Could you check a few things on this model? Use its own coordinates, in mm. A direction names the side the tool comes from. Round coordinates to 2 decimals unless told otherwise and drop trailing zeros. Loops run counter-clockwise (first coordinate to the right, second up) from the corner with the lowest first, then second, coordinate; pieces in that order, holes last. Notation, with made-up numbers: (89, 42.25) -> (124, 42.25) arc R28 cw to (124, 78.25) -> close; hole circle Ø4 at (3.5, -9.5). An arc over 180 degrees is marked (long way). One line per item, written item: value.
from build123d import *

# Parameters (mm, degrees)
F0_R     = 10.5
F0_W     = 6
F0_H     = 27
F0_W_2   = 3
F1_DEPTH = 3
F2_DEPTH = 22
F3_R     = 2.99999
F5_R     = 10.5
F6_DEPTH = 12
F7_DEPTH = 3
F8_R     = 5


# Not quite as in the source:
# - a fillet or chamfer is up to 0.001 mm smaller than in the source, because OpenCascade refuses the exact size


with BuildPart() as f1:
    # F0 (on Top) → F1 (new body)
    with BuildSketch(Plane.XY):
        with BuildLine():
            ThreePointArc((0, -13.5), (9.545941546, -9.545941546), (13.5, 0))
            ThreePointArc((13.5, 0), (9.545941546, 9.545941546), (0, 13.5))
            ThreePointArc((0, 13.5), (-13.5, 0), (0, -13.5))
        make_face()
        Circle(F0_R, mode=Mode.SUBTRACT)
        with BuildLine():
            Line((13.5, -13.5), (13.5, 0))
            ThreePointArc((13.5, 0), (9.545941546, -9.545941546), (0, -13.5))
            Line((0, -13.5), (13.5, -13.5))
        make_face()
        with BuildLine():
            ThreePointArc((0, 13.5), (9.545941546, 9.545941546), (13.5, 0))
            Line((13.5, 0), (13.5, 13.5))
            Line((13.5, 13.5), (0, 13.5))
        make_face()
        Polygon((13.5, 13.5), (13.5, 0), (13.5, -13.5), (16.5, -13.5), (16.5, 13.5), align=None)
        with Locations((19.5, 0)):
            Rectangle(F0_W, F0_H)
        with Locations((24, 0)):
            Rectangle(F0_W_2, F0_H)
    extrude(amount=F1_DEPTH)

    # F0 (on Top) → F2 (join)
    with BuildSketch(Plane.XY):
        with BuildLine():
            ThreePointArc((0, -13.5), (9.545941546, -9.545941546), (13.5, 0))
            ThreePointArc((13.5, 0), (9.545941546, 9.545941546), (0, 13.5))
            ThreePointArc((0, 13.5), (-13.5, 0), (0, -13.5))
        make_face()
        Circle(F0_R, mode=Mode.SUBTRACT)
        with BuildLine():
            ThreePointArc((0, 13.5), (9.545941546, 9.545941546), (13.5, 0))
            Line((13.5, 0), (13.5, 13.5))
            Line((13.5, 13.5), (0, 13.5))
        make_face()
        Polygon((13.5, 13.5), (13.5, 0), (13.5, -13.5), (16.5, -13.5), (16.5, 13.5), align=None)
        with Locations((24, 0)):
            Rectangle(F0_W_2, F0_H)
        with BuildLine():
            Line((13.5, -13.5), (13.5, 0))
            ThreePointArc((13.5, 0), (9.545941546, -9.545941546), (0, -13.5))
            Line((0, -13.5), (13.5, -13.5))
        make_face()
    extrude(amount=-F2_DEPTH)

    # F3 (radius 3 in the source; OpenCascade refuses exactly that, so slightly less here)
    f3_edges = [f1.edges().sort_by_distance(p)[0] for p in [
        (16.5, 0, 0),
        (22.5, 0, 0),
        (25.5, 0, 3),
    ]]
    fillet(f3_edges, radius=F3_R)



with BuildPart() as f6:
    # F5 (on offset) → F6 (new body)
    with BuildSketch(Plane(origin=(0, 0, -10), x_dir=(1, 0, 0), z_dir=(0, 0, -1))):
        with BuildLine():
            Line((16.5, 13.5), (0, 13.5))
            ThreePointArc((0, 13.5), (-13.5, 0), (0, -13.5))
            Line((0, -13.5), (16.5, -13.5))
            Line((16.5, -13.5), (16.5, 13.5))
        make_face()
        Circle(F5_R, mode=Mode.SUBTRACT)
    extrude(amount=-F6_DEPTH)


with BuildPart() as f1_1:
    add(f1.part)

    add(f6.part)  # F7 merges F6
    # F5 (on offset) → F7 (join)
    with BuildSketch(Plane(origin=(0, 0, -10), x_dir=(1, 0, 0), z_dir=(0, 0, -1))):
        with BuildLine():
            Line((16.5, 13.5), (0, 13.5))
            ThreePointArc((0, 13.5), (-13.5, 0), (0, -13.5))
            Line((0, -13.5), (16.5, -13.5))
            Line((16.5, -13.5), (16.5, 13.5))
        make_face()
        Circle(F5_R, mode=Mode.SUBTRACT)
        with BuildLine():
            ThreePointArc((0, -13.5), (-13.5, 0), (0, 13.5))
            Line((0, 13.5), (-43.5, 13.5))
            Line((-43.5, 13.5), (-43.5, 4))
            Line((-43.5, 4), (-28.5, 4))
            ThreePointArc((-28.5, 4), (-24.5, 0), (-28.5, -4))
            Line((-28.5, -4), (-43.5, -4))
            Line((-43.5, -4), (-43.5, -13.5))
            Line((-43.5, -13.5), (0, -13.5))
        make_face()
    extrude(amount=F7_DEPTH)

    # F8
    f8_edges = [f1_1.edges().sort_by_distance(p)[0] for p in [
        (-43.5, -13.5, -11.5),
        (-43.5, 13.5, -11.5),
    ]]
    fillet(f8_edges, radius=F8_R)


solid = f1_1.part
(1) If we section it at C-C, the plane z = -13.75: Please give me the cut outline in (x, y).
Recorded:
outline: (0, -13.5) -> (16.5, -13.5) -> (16.5, 13.5) -> (0, 13.5) arc R13.5 ccw to start; (22.5, -13.5) -> (25.5, -13.5) -> (25.5, 13.5) -> (22.5, 13.5) -> close; hole circle Ø21 at (0, 0)
(2) If I drill on L1, parallel to Y at x = 0, z = -5.25; L2, parallel to X at y = -8.25, z = -12; L3, parallel to X at y = 6.25, z = -2, over which ranges is the centre line in solid material (lowest first)?
Recorded:
L1: -13.5 to -10.5, 10.5 to 13.5
L2: -43.5 to -6.5, 6.5 to 16.5, 22.5 to 25.5
L3: -11.97 to -8.44, 8.44 to 16.67, 22.33 to 25.5
(3) I'm going to push flat-ended pins straight in: pin 1 Ø2 at (x, y) = (-11.5, 11) entering from -Z; pin 2 Ø10 at (x, y) = (-27.5, 6.5) entering from +Z. Where does each tip first touch, or does it pass through?
Recorded:
pin 1: z = -13
pin 2: z = -10
(4) Thinking about a two-plate mould opening in Y: for faces 4 (the face through (0.2, -13.5, -9.3)), 5 (the face through (-43.5, 6, -11)), 6 (the face through (-36, -4, -11)), which applies, released by +Y, released by -Y, zero draft, split by the parting line, or undercut?
Recorded:
face 4: released by -Y
face 5: zero draft
face 6: undercut
(5) If we section it at A-A, the plane x = -34: Please give me the cut outline in (y, z), then the cut area to 3 significant figures.
Recorded:
outline: (-13.5, -13) -> (-4, -13) -> (-4, -10) -> (-13.5, -10) -> close; (4, -13) -> (13.5, -13) -> (13.5, -10) -> (4, -10) -> close
area: 57.0 mm²
(6) For faces 1 (the face through (-13.497, -0.297, -17.563)), 2 (the face through (-13.497, -0.297, -3.591)), 3 (the face through (22.5, 0, -12)), which set-ups out of +Z, -Z, +X, -X, +Y, -Y let a thin tool reach every point of the face, with its end or its side?
Recorded:
face 1: -Z, -X
face 2: +Z, -X
face 3: -Z, +Y, -Y
